Source: CAD feature listing. Evaluate the final solid. Frame: model axes, mm. Coordinates: 2 decimals unless noted, no trailing zeros. Write each loop counter-clockwise with the first axis right and the second up, starting at its lowest first coordinate (ties: lowest second). Pieces come first, ordered by that corner, then holes. Notation, with made-up numbers: (-34.75, 66) - (-16.75, 66) arc R20 ccw to (-16.75, 93) - close; hole circle Ø1 at (21, -24.75). An arc over 180 degrees is marked (long way). One line per question, with ' | ' between items. Start each with the question number.
Q1. Contact query for flat-ended pins moving along their axis: P1, Ø1.5, axis at y = 3.5, z = 4.5, coming from the +X side; P2, Ø1, axis at x = 1, z = 3.5, coming from the -Y side; P3, Ø6, axis at x = -12.5, z = 3, coming from the +Y side; P4, Ø1, axis at x = 3, y = 20.5, coming from the -Z side. Output: stop coordinate, or through.
Q2. Cut plane A-A, the plane z = 9.25. Return loops of the section in (x, y).
Q3. Line query: line 1 (Z direction, x = -18, y = 15); line 2 (Y direction, x = -18.5, z = 3); line 3 (X direction, y = 1, z = 2). Output: solid intervals per line, ascending.
Q4. Cut plane B-B, the plane z = 3. Return loops of the section in (x, y).
```python
from build123d import *

# Parameters (mm, degrees)
F1_DEPTH = 10
F0_R     = 29.217715
F2_DEPTH = 4
F3_R     = 2
F4_DEPTH = 4


with BuildPart() as f1:
    # F0 (on Top) → F1 (new body)
    with BuildSketch(Plane.XY):
        with BuildLine():
            ThreePointArc((0.009298, -19.999998), (-20, -0.000754), (0.007791, 19.999998))
            Line((0.007791, 19.999998), (0.00857, 21.999998))
            ThreePointArc((0.00857, 21.999998), (-22, -0.000829), (0.010228, -21.999998))
            Line((0.010228, -21.999998), (0.009298, -19.999998))
        make_face()
    extrude(amount=F1_DEPTH)

    # F0 (on Top) → F2 (join)
    with BuildSketch(Plane.XY):
        Circle(F0_R)
        with BuildLine():
            ThreePointArc((0.010228, -21.999998), (-22, -0.000829), (0.00857, 21.999998))
            ThreePointArc((0.00857, 21.999998), (15.559379, 15.553319), (22, 0))
            ThreePointArc((22, 0), (15.559965, -15.552733), (0.010228, -21.999998))
        make_face(mode=Mode.SUBTRACT)
    extrude(amount=F2_DEPTH)

    # F3
    f3_edges = [f1.edges().sort_by_distance(p)[0] for p in [
        (-29.217715, 0, 4),
    ]]
    fillet(f3_edges, radius=F3_R)

    # F0 (on Top) → F4 (join)
    with BuildSketch(Plane.XY):
        with BuildLine():
            ThreePointArc((0.007791, 19.999998), (14.14489, 14.139381), (20, 0))
            ThreePointArc((20, 0), (14.145423, -14.138848), (0.009298, -19.999998))
            Line((0.009298, -19.999998), (0.010228, -21.999998))
            ThreePointArc((0.010228, -21.999998), (15.559965, -15.552733), (22, 0))
            ThreePointArc((22, 0), (15.559379, 15.553319), (0.00857, 21.999998))
            Line((0.00857, 21.999998), (0.007791, 19.999998))
        make_face()
    extrude(amount=F4_DEPTH)


solid = f1.part
```
Reply:
1) P1: stops at x = 27.97 | P2: stops at y = -28.93 | P3: stops at y = 27.58 | P4: stops at z = 0
2) outline: (0.01, -22) - (0.01, -20) arc R20 cw to (0.01, 20) - (0.01, 22) arc R22 ccw to start
3) line 1: z = 0 to 4 | line 2: y = -22.27 to -7.6, 7.6 to 22.27 | line 3: x = -29.2 to -19.97, 19.97 to 29.2
4) outline: circle Ø57.9 at (0, 0); hole (0.01, 20) arc R20 ccw (long way) to (20, 0) arc R20 ccw to start
